The drawing under review shows one solid part. Ordinate dimensions are in mm from its lowest x, y, z. Round coordinates to 2 decimals unless told otherwise and drop trailing zeros. Order: outer loops, then holes, each group sorted by start corner. A loop starts at its lowest first (then second) coordinate and runs counter-clockwise, first axis right, second up. Notation, with made-up numbers: (64.25, 40) - (78.25, 40) arc R16 cw to (78.25, 45) - close; hole circle Ø11 at (-9, 70). An arc over 180 degrees is marked (long way). One line per question, with ' | ' between items.
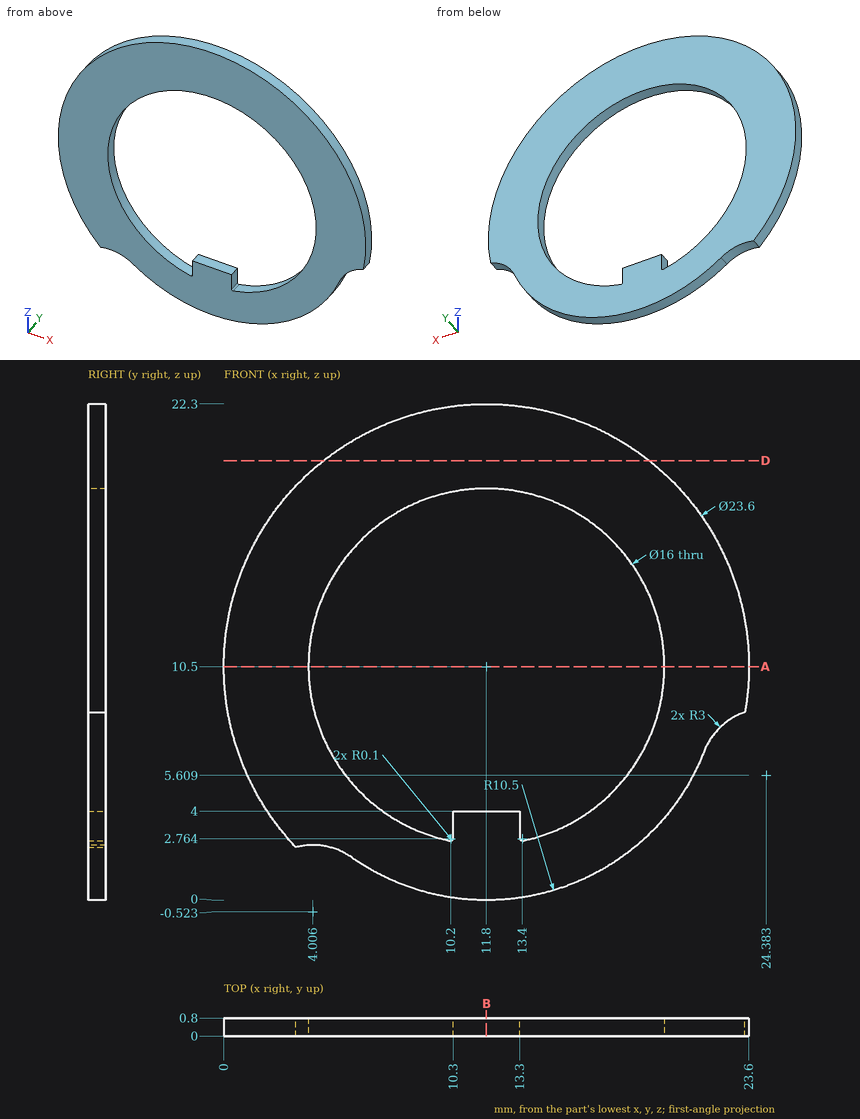
(1) We need section A-A on z = 10.5. State the section outline as (x, y) points.
Output values:
outline: (0, 0) - (3.8, 0) - (3.8, 0.8) - (0, 0.8) - close; (19.8, 0) - (23.6, 0) - (23.6, 0.8) - (19.8, 0.8) - close
(2) Insertion check: pin 1 (8 mm diameter, centred on x = 10.5, z = 5.5, fed in from +Y); pin 2 (4 mm diameter, centred on x = 8, z = 7.5, fed in from -Y). Each pin has a flat end and moves straight along its axis. Give the tip position at first contact, or say it passes through.
Output values:
pin 1: y = 0.8 | pin 2: through
(3) We need section D-D on z = 19.75. State the section outline as (x, y) points.
Output values:
outline: (4.47, 0) - (19.13, 0) - (19.13, 0.8) - (4.47, 0.8) - close
(4) For probe 1 along Z at (x, y) = (11.8, 0.25); probe 2 along X at (y, z) = (0.2, 10.5); probe 3 along X at (y, z) = (0.4, 3.5) (1 decimal), list the stretches that pass through material, from the lowest coordinate up. Write a range as [from, to].
Output values:
probe 1: [0, 4], [18.5, 22.3] | probe 2: [0, 3.8], [19.8, 23.6] | probe 3: [2.3, 7.9], [10.3, 13.3], [15.7, 19.6]
(5) We need section B-B on x = 11.8. State the section outline as (y, z) points.
Output values:
outline: (0, 0) - (0.8, 0) - (0.8, 4) - (0, 4) - close; (0, 18.5) - (0.8, 18.5) - (0.8, 22.3) - (0, 22.3) - close
